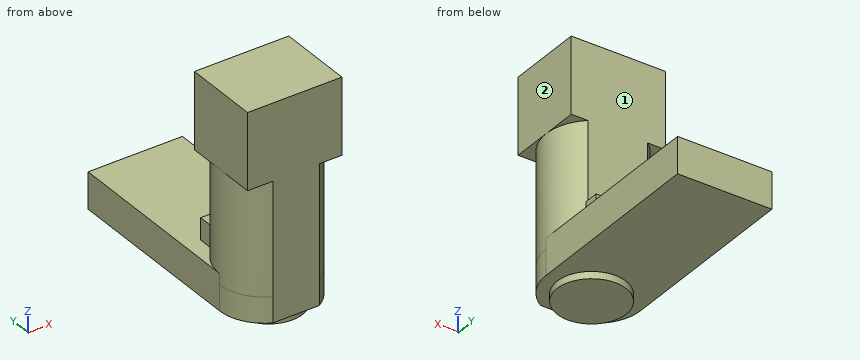
from build123d import *

# Parameters (mm, degrees)
SKETCH2_W            = 13
SKETCH2_H            = 11.1
SKETCH2_W_2          = 12.5
SKETCH2_H_2          = 10.6
BOSS_EXTRUDE1_DEPTH  = 10
SKETCH3_W            = 12.5
SKETCH3_H            = 10.6
BOSS_EXTRUDE2_DEPTH  = 10
BOSS_EXTRUDE3_DEPTH  = 15.5
BOSS_EXTRUDE4_DEPTH  = 1.5
BOSS_EXTRUDE5_DEPTH  = 3.52
SKETCH9_W            = 13
SKETCH9_H            = 11.1
BOSS_EXTRUDE7_DEPTH  = 0.5
SKETCH10_W           = 24.5
SKETCH10_H           = 0.6
CUT_EXTRUDE1_DEPTH   = 15
BOSS_EXTRUDE8_DEPTH  = 3
SKETCH13_R           = 4.75
BOSS_EXTRUDE9_DEPTH  = 0.98
SKETCH15_W           = 13
SKETCH15_H           = 5.02
BOSS_EXTRUDE11_DEPTH = 15


with BuildPart() as part:
    # Sketch2 → Boss-Extrude1 (new body)
    with BuildSketch(Plane.XY):
        Rectangle(SKETCH2_W, SKETCH2_H)
        Rectangle(SKETCH2_W_2, SKETCH2_H_2, mode=Mode.SUBTRACT)
    extrude(amount=BOSS_EXTRUDE1_DEPTH)

    # Sketch3 → Boss-Extrude2 (add)
    with BuildSketch(Plane(origin=(0, 0, 0), x_dir=(-1, 0, 0), z_dir=(0, 0, -1))):
        Rectangle(SKETCH3_W, SKETCH3_H)
    extrude(amount=-BOSS_EXTRUDE2_DEPTH)

    # Sketch4 → Boss-Extrude3 (add)
    with BuildSketch(Plane(origin=(0, 0, 0), x_dir=(-1, 0, 0), z_dir=(0, 0, -1))):
        with BuildLine():
            Line((-3.383415434, -5.55), (2.983923173, -5.55))
            ThreePointArc((2.983923173, -5.55), (6.5, 0), (2.983923173, 5.55))
            Line((2.983923173, 5.55), (-3.383415434, 5.55))
            ThreePointArc((-3.383415434, 5.55), (-6.5, 0), (-3.383415434, -5.55))
        make_face()
    extrude(amount=BOSS_EXTRUDE3_DEPTH)

    # Sketch5 → Boss-Extrude4 (add)
    with BuildSketch(Plane(origin=(0, 0, -15.5), x_dir=(-1, 0, 0), z_dir=(0, 0, -1))):
        with BuildLine():
            Line((6.5, 0), (-6.5, 0))
            ThreePointArc((-6.5, 0), (-5.667547985, -3.182593257), (-3.383415434, -5.55))
            Line((-3.383415434, -5.55), (2.983923173, -5.55))
            ThreePointArc((2.983923173, -5.55), (5.547001926, -3.285015078), (6.5, 0))
        make_face()
        with BuildLine():
            Line((6.5, 10.96), (-6.5, 10.96))
            Line((-6.5, 10.96), (-6.5, 0))
            ThreePointArc((-6.5, 0), (-5.667547985, 3.182593257), (-3.383415434, 5.55))
            Line((-3.383415434, 5.55), (2.983923173, 5.55))
            ThreePointArc((2.983923173, 5.55), (5.547001926, 3.285015078), (6.5, 0))
            Line((6.5, 0), (6.5, 10.96))
        make_face()
    extrude(amount=-BOSS_EXTRUDE4_DEPTH)

    # Sketch6 → Boss-Extrude5 (add)
    with BuildSketch(Plane(origin=(0, 0, -15.5), x_dir=(-1, 0, 0), z_dir=(0, 0, -1))):
        with BuildLine():
            Line((-6.5, 0), (-6.5, 10.96))
            Line((-6.5, 10.96), (6.5, 10.96))
            Line((6.5, 10.96), (6.5, 0))
            ThreePointArc((6.5, 0), (5.547001926, -3.285015078), (2.983923173, -5.55))
            Line((2.983923173, -5.55), (-3.383415434, -5.55))
            ThreePointArc((-3.383415434, -5.55), (-5.667547985, -3.182593257), (-6.5, 0))
        make_face()
    extrude(amount=BOSS_EXTRUDE5_DEPTH)

    # Sketch9 → Boss-Extrude7 (add)
    with BuildSketch(Plane.XY.offset(10)):
        Rectangle(SKETCH9_W, SKETCH9_H)
    extrude(amount=BOSS_EXTRUDE7_DEPTH)

    # Sketch10 → Cut-Extrude1 (cut)
    with BuildSketch(Plane.ZY.offset(6.5)):
        with Locations((-1.75, 5.25)):
            Rectangle(SKETCH10_W, SKETCH10_H)
    extrude(amount=-CUT_EXTRUDE1_DEPTH, mode=Mode.SUBTRACT)

    # Sketch11 → Boss-Extrude8 (add)
    with BuildSketch(Plane.XY.offset(-14)):
        Polygon((-3.991590331, 4.95), (0.110593925, 4.95), (0.110593925, 6.95), (-4.241590331, 6.95), (-4.241590331, 4.95), align=None)
        Polygon((4.212778181, 4.95), (4.462778181, 4.95), (4.462778181, 6.95), (0.110593925, 6.95), (0.110593925, 4.95), align=None)
    extrude(amount=BOSS_EXTRUDE8_DEPTH)

    # Sketch13 → Boss-Extrude9 (add)
    with BuildSketch(Plane(origin=(0, 0, -19.02), x_dir=(-1, 0, 0), z_dir=(0, 0, -1))):
        with Locations((-0.048060538, -0.29)):
            Circle(SKETCH13_R)
    extrude(amount=BOSS_EXTRUDE9_DEPTH)

    # Sketch15 → Boss-Extrude11 (add)
    with BuildSketch(Plane(origin=(0, 10.96, 0), x_dir=(1, 0, 0), z_dir=(0, 1, 0))):
        with Locations((0, 16.51)):
            Rectangle(SKETCH15_W, SKETCH15_H)
    extrude(amount=BOSS_EXTRUDE11_DEPTH)


solid = part.part
The model under review builds one solid part; all positions refer to its coordinate system, in mm. Face numbers are marked on the shaded views. A direction names the side the tool comes from. Give positions to 0.01 mm unless a question says otherwise; leave off trailing zeros. Loops run counter-clockwise (first coordinate to the right, second up) from the corner with the lowest first, then second, coordinate; pieces in that order, holes last. Notation, with made-up numbers: (7.25, -39) -> (13.25, -39) arc R16 ccw to (13.25, -8) -> close; hole circle Ø7 at (63.5, 71.25). An arc over 180 degrees is marked (long way). Write each question's results on one line, items separated by ' | '.
1) Take a section at A-A, the plane z = -12.5. Give the boundary of the cut face in (x, y), plus the area to 3 significant figures.
Conclusion:
outline: (-4.24, 4.95) -> (-3.99, 4.95) arc R6.14 ccw to (-2.98, -5.55) -> (3.38, -5.55) arc R6.5 ccw to (4.21, 4.95) -> (4.46, 4.95) -> (4.46, 6.95) -> (-4.24, 6.95) -> close | area: 136 mm^2
2) Take a section at B-B, the plane y = -2.5. Give the boundary of the cut face in (x, z).
Conclusion:
outline: (-6.5, 0) -> (-5.97, 0) -> (-5.97, -19.02) -> (-4.16, -19.02) -> (-4.16, -20) -> (4.25, -20) -> (4.25, -19.02) -> (6, -19.02) -> (6, 0) -> (6.5, 0) -> (6.5, 10.5) -> (-6.5, 10.5) -> close
3) Take a section at C-C, the plane x = 0.5. Give the boundary of the cut face in (y, z).
Conclusion:
outline: (-5.55, -19.02) -> (-5.02, -19.02) -> (-5.02, -20) -> (4.44, -20) -> (4.44, -19.02) -> (25.96, -19.02) -> (25.96, -14) -> (6.95, -14) -> (6.95, -11) -> (4.95, -11) -> (4.95, 10.5) -> (-5.55, 10.5) -> close
4) Take a section at D-D, the plane z = -17. Give the boundary of the cut face in (x, y).
Conclusion:
outline: (-6.5, 0) arc R6.14 ccw to (-2.98, -5.55) -> (3.38, -5.55) arc R6.5 ccw to (6.5, 0) -> (6.5, 25.96) -> (-6.5, 25.96) -> close
5) Insertion check: pin 1 Ø12 at (y, z) = (5, 4.5) entering from -X; pin 2 Ø1.1 at (x, y) = (-5, -2.5) entering from -Z; pin 3 Ø1 at (y, z) = (5.5, -12) entering from +X; pin 4 Ø1.6 at (x, y) = (2, 6.5) entering from +Z. Each pin has a flat end and moves straight along its axis. Give the tip position at first contact, or say it passes through.
Conclusion:
pin 1: stops at x = -6.5 | pin 2: stops at z = -19.02 | pin 3: stops at x = 4.46 | pin 4: stops at z = -11
6) Tool access review of the marked faces 1 and 2: name each direction out of +Z, -Z, +X, -X, +Y, -Y from which nothing blocks a thin tool from reaching the whole face with its end or side.
Conclusion:
face 1: +Z, +X, -X, +Y | face 2: +Z, -Z, +X, +Y, -Y
7) For line 1 along Z through (x, y) = (5.75, 3.5); line 2 along Z through (x, y) = (-0.75, 14); line 3 along Z through (x, y) = (0.75, 6), list the stretches that pass through material, from the lowest coordinate up. Write a range as from..to.
Conclusion:
line 1: z = -19.02..-14, 0..10.5 | line 2: z = -19.02..-14 | line 3: z = -19.02..-11
